Part print with two shaded views. Sizes in mm from the minimum x, y, z corner. A direction names the side the tool comes from. Round coordinates to 2 decimals unless told otherwise and drop trailing zeros. Order: outer loops, then holes, each group sorted by start corner. A loop starts at its lowest first (then second) coordinate and runs counter-clockwise, first axis right, second up. Notation, with made-up numbers: (-9.5, 63.25) - (44.5, 63.25) arc R21 ccw to (44.5, 87.25) - close; hole circle Ø10 at (16, 83.5). An arc over 180 degrees is marked (long way). Use one line per item in the form item = value.
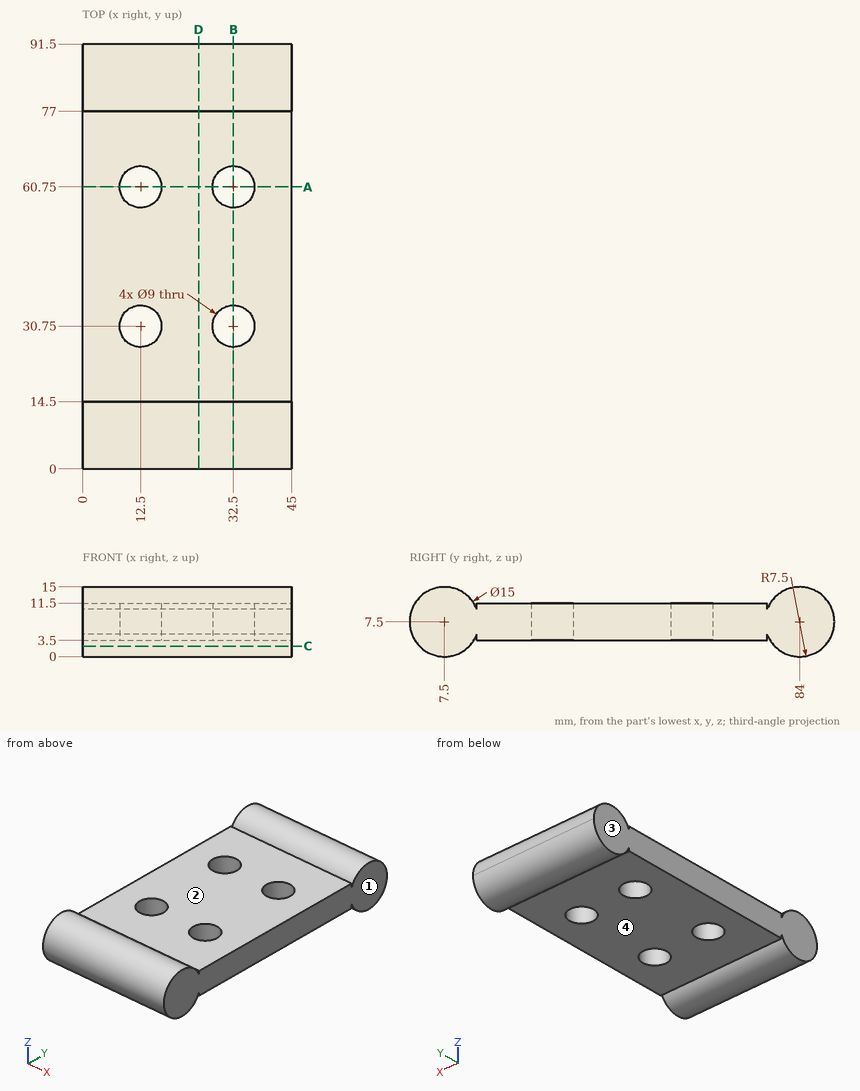
(1) Slice it at C-C on z = 2.25. Give the cut face in (x, y).
Report:
outline = (0, 2.14) - (45, 2.14) - (45, 12.86) - (0, 12.86) - close; (0, 78.64) - (45, 78.64) - (45, 89.36) - (0, 89.36) - close
(2) Tool access for the marked faces 1 and 2: list every direction of +Z, -Z, +X, -X, +Y, -Y with a clear straight run to the whole face (end or side of a thin tool).
Report:
face_1 = +Z, -Z, +X, +Y, -Y
face_2 = +Z, +X, -X
(3) Slice it at B-B on x = 32.5. Give the cut face in (y, z), then the cut area to 3 significant figures.
Report:
outline = (14.5, 3.5) - (26.25, 3.5) - (26.25, 11.5) - (14.5, 11.5) - (14.5, 10.19) arc R7.5 ccw (long way) to (14.5, 4.81) - close; (35.25, 3.5) - (56.25, 3.5) - (56.25, 11.5) - (35.25, 11.5) - close; (65.25, 3.5) - (77, 3.5) - (77, 4.81) arc R7.5 ccw (long way) to (77, 10.19) - (77, 11.5) - (65.25, 11.5) - close
area = 706 mm2
(4) Slice it at D-D on x = 25. Give the cut face in (y, z), then the cut area to 3 significant figures.
Report:
outline = (14.5, 3.5) - (77, 3.5) - (77, 4.81) arc R7.5 ccw (long way) to (77, 10.19) - (77, 11.5) - (14.5, 11.5) - (14.5, 10.19) arc R7.5 ccw (long way) to (14.5, 4.81) - close
area = 850 mm2
(5) Probe probe 1 along Y at (x, z) = (12.5, 7); probe 2 along Y at (x, z) = (30, 9.75); probe 3 along Y at (x, z) = (32.5, 11). List the from-to ranges inside material, lowest first. Write a range as [from, to].
Report:
probe_1 = [0.02, 26.25], [35.25, 56.25], [65.25, 91.48]
probe_2 = [0.35, 27.01], [34.49, 57.01], [64.49, 91.15]
probe_3 = [0.87, 14.13], [14.5, 26.25], [35.25, 56.25], [65.25, 77], [77.37, 90.63]
(6) Slice it at A-A on y = 60.75. Give the cut face in (x, z).
Report:
outline = (0, 3.5) - (8, 3.5) - (8, 11.5) - (0, 11.5) - close; (17, 3.5) - (28, 3.5) - (28, 11.5) - (17, 11.5) - close; (37, 3.5) - (45, 3.5) - (45, 11.5) - (37, 11.5) - close
(7) Pin check, flat tips, straight feed: pin 1 (1.4 mm diameter, centred on x = 21, z = 11, fed in from -Y); pin 2 (10 mm diameter, centred on x = 28.5, y = 66, fed in from +Z); pin 3 (1 mm diameter, centred on x = 24, z = 4, fed in from +Y). Stop position of each tip, or through.
Report:
pin_1 = 0.54
pin_2 = 11.5
pin_3 = 90.87
(8) Pull direction Y, two halves, no side cores. Call the marked faces 3 and 4: released by +Y, released by -Y, zero draft, split by the parting line, or undercut.
Report:
face_3 = zero draft
face_4 = undercut
